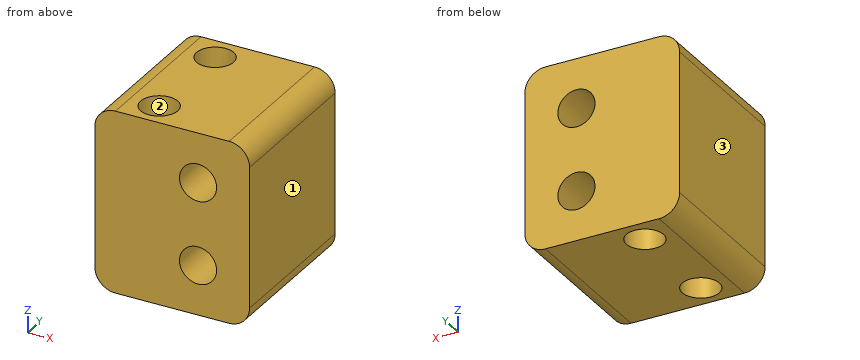
```python
from build123d import *

# Parameters (mm, degrees)
SKETCH1_W           = 19.05
SKETCH1_H           = 22.352
SKETCH1_R           = 2.286
BOSS_EXTRUDE1_DEPTH = 19.05
FILLET1_R           = 2.54
FILLET2_R           = 2.54
SKETCH2_R           = 2.286
CUT_EXTRUDE1_DEPTH  = 31.874585487


with BuildPart() as part:
    # Sketch1 → Boss-Extrude1 (new body)
    with BuildSketch(Plane(origin=(0, 0, 0), x_dir=(1, 0, 0), z_dir=(0, 1, 0))):
        Rectangle(SKETCH1_W, SKETCH1_H)
        with Locations(Location((3.175, 5.08, 0), (0, 0, 90))):
            Circle(SKETCH1_R, mode=Mode.SUBTRACT)
        with Locations(Location((3.175, -5.08, 0), (0, 0, 90))):
            Circle(SKETCH1_R, mode=Mode.SUBTRACT)
    extrude(amount=BOSS_EXTRUDE1_DEPTH)

    # Fillet1
    fillet1_edges = [part.edges().sort_by_distance(p)[0] for p in [
        (9.525, 9.525, 11.176),
        (9.525, 9.525, -11.176),
    ]]
    fillet(fillet1_edges, radius=FILLET1_R)

    # Fillet2
    fillet2_edges = [part.edges().sort_by_distance(p)[0] for p in [
        (-9.525, 9.525, 11.176),
        (-9.525, 9.525, -11.176),
    ]]
    fillet(fillet2_edges, radius=FILLET2_R)

    # Sketch2 → Cut-Extrude1 (cut, through all)
    with BuildSketch(Plane.XY.offset(11.176)):
        with Locations((-3.429, 15.748)):
            Circle(SKETCH2_R)
        with Locations(Location((-3.429, 3.302, 0), (0, 0, 180))):
            Circle(SKETCH2_R)
    extrude(amount=-CUT_EXTRUDE1_DEPTH, mode=Mode.SUBTRACT)


solid = part.part
```
The model under review builds one solid part; all positions refer to its coordinate system, in mm. Face numbers are marked on the shaded views. Round coordinates to 2 decimals unless told otherwise and drop trailing zeros. Loops run counter-clockwise (first coordinate to the right, second up) from the corner with the lowest first, then second, coordinate; pieces in that order, holes last. Notation, with made-up numbers: (3.5, 71.5) - (45.5, 71.5) arc R16 cw to (45.5, 102.5) - close; hole circle Ø9 at (-34.5, 76). An arc over 180 degrees is marked (long way). Use a Markdown table: item, result. Add a question column.
Q1. Add section D-D (y = 17.5). State the section outline as (x, z) points (3 decimals), plus the area to 3 significant figures.
Q2. Add section B-B (z = -7). State the section outline as (x, y) points (3 decimals), plus the area to 3 significant figures.
Q3. The part is to be moulded in two halves that separate along X. For the marked faces 1, 2 and 3, say which applies: pulls with the +X half, pulls with the -X half, needs draft (parallel to the pull), parting line crosses it, or undercut.
Q4. Add section A-A (y = 14.25). State the section outline as (x, z) points (3 decimals), plus the area to 3 significant figures.
Q5. For probe 1 along Z at (x, y) = (3.25, 9); probe 2 along Y at (x, z) = (-5.5, 3.75); probe 3 along Y at (x, z) = (-4.75, -2.5), list the stretches that pass through material, from the lowest coordinate up.
Q6. Add section C-C (x = 2.75). State the section outline as (y, z) points, plus the area to 3 significant figures.
Worked answers:
| question | item | result |
|---|---|---|
| 1 | outline | (-9.525, -8.636) arc R2.54 ccw to (-6.985, -11.176) - (-4.897, -11.176) - (-4.897, 11.176) - (-6.985, 11.176) arc R2.54 ccw to (-9.525, 8.636) - close; (-1.961, -11.176) - (6.985, -11.176) arc R2.54 ccw to (9.525, -8.636) - (9.525, 8.636) arc R2.54 ccw to (6.985, 11.176) - (-1.961, 11.176) - close; hole circle Ø4.572 at (3.175, -5.08); hole circle Ø4.572 at (3.175, 5.08) |
| 1 | area | 322 mm² |
| 2 | outline | (-9.525, 0) - (1.934, 0) - (1.934, 19.05) - (-9.525, 19.05) - close; (4.416, 0) - (9.525, 0) - (9.525, 19.05) - (4.416, 19.05) - close; hole circle Ø4.572 at (-3.429, 3.302); hole circle Ø4.572 at (-3.429, 15.748) |
| 2 | area | 283 mm² |
| 3 | face 1 | pulls with the +X half |
| 3 | face 2 | undercut |
| 3 | face 3 | pulls with the -X half |
| 4 | outline | (-9.525, -8.636) arc R2.54 ccw to (-6.985, -11.176) - (-5.156, -11.176) - (-5.156, 11.176) - (-6.985, 11.176) arc R2.54 ccw to (-9.525, 8.636) - close; (-1.702, -11.176) - (6.985, -11.176) arc R2.54 ccw to (9.525, -8.636) - (9.525, 8.636) arc R2.54 ccw to (6.985, 11.176) - (-1.702, 11.176) - close; hole circle Ø4.572 at (3.175, -5.08); hole circle Ø4.572 at (3.175, 5.08) |
| 4 | area | 310 mm² |
| 5 | probe 1 | -11.18 to -7.36, -2.8 to 2.8, 7.36 to 11.18 |
| 5 | probe 2 | 0 to 2.33, 4.27 to 14.78, 16.72 to 19.05 |
| 5 | probe 3 | 0 to 1.44, 5.17 to 13.88, 17.61 to 19.05 |
| 6 | outline | (0, -11.18) - (19.05, -11.18) - (19.05, -7.33) - (0, -7.33) - close; (0, -2.83) - (19.05, -2.83) - (19.05, 2.83) - (0, 2.83) - close; (0, 7.33) - (19.05, 7.33) - (19.05, 11.18) - (0, 11.18) - close |
| 6 | area | 255 mm² |
